Here's how the part is built. I have some questions about the finished solid (model axes, mm). Give positions to 0.01 mm unless a question says otherwise; leave off trailing zeros. Write each loop counter-clockwise with the first axis right and the second up, starting at its lowest first coordinate (ties: lowest second). Pieces come first, ordered by that corner, then holes. Notation, with made-up numbers: M -17,-33.5 L -8,-33.5 A13 ccw -8,-20.5 Z; hole C 85,54.25 d11. An arc over 180 degrees is marked long. Answer as CSV lines item,"result". Start each with the question number.
Q1. Suppose I cut it at A-A (z = 5.75). Write out the boundary of the cut face in (x, y).
Q2. If I drill on line 1 along Y through (x, z) = (-19.5, 3.25); line 2 along Y through (x, z) = (53, 0.5); line 3 along X through (y, z) = (13, 4), over which ranges is the centre line in solid material (lowest first)?
Q3. For pin 1 (5 mm diameter, centred on y = 28.5, z = 7.5, fed in from +X); pin 2 (3 mm diameter, centred on x = -25, z = 3.5, fed in from -Y); pin 3 (3 mm diameter, centred on y = 19, z = 2, fed in from -X), each with a flat end and sliding along its axis, tell me the tip position at first contact or that it passes through.
```python
from build123d import *

# Parameters (mm, degrees)
EXTRUDE_1_DEPTH = 10
FILLET_1_R      = 0.5


with BuildPart() as part:
    # 草图1 → 凸台-拉伸1 (new body)
    with BuildSketch(Plane.XY):
        Polygon((-37.5, 37.5), (37.5, 37.5), (75, 0), (0, 0), align=None)
    extrude(amount=EXTRUDE_1_DEPTH)

    # 圆角1
    fillet_1_edges = [part.edges().sort_by_distance(p)[0] for p in [
        (0, 37.5, 10),
        (-18.75, 18.75, 10),
        (37.5, 0, 10),
        (-18.75, 18.75, 0),
        (0, 37.5, 0),
        (56.25, 18.75, 0),
        (37.5, 0, 0),
        (56.25, 18.75, 10),
        (0, 0, 5),
        (-37.5, 37.5, 5),
        (37.5, 37.5, 5),
        (75, 0, 5),
    ]]
    fillet(fillet_1_edges, radius=FILLET_1_R)


solid = part.part
```
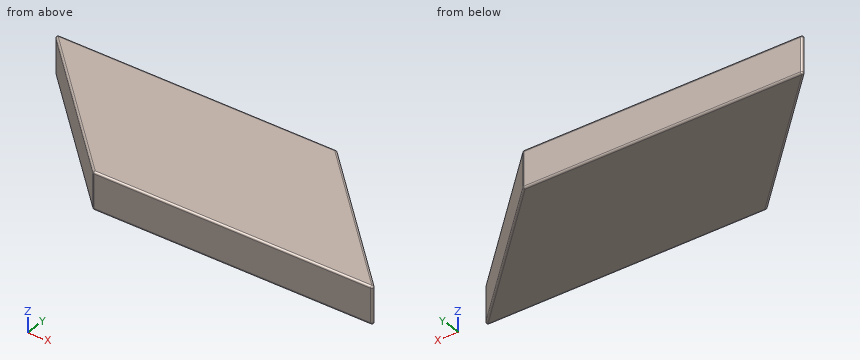
Resolved:
1,outline,"M -36.65,36.65 L -0.15,0.15 A0.5 ccw 0.21,0 L 73.79,0 A0.5 ccw 74.15,0.85 L 37.65,37.35 A0.5 ccw 37.29,37.5 L -36.29,37.5 A0.5 ccw Z"
2,line 1,"19.5 to 37.5"
2,line 2,"0 to 22"
2,line 3,"-13 to 62"
3,pin 1,"x = 49"
3,pin 2,"y = 23.5"
3,pin 3,"x = -20.5"
